The drawing under review shows one solid part. Ordinate dimensions are in mm from its lowest x, y, z. Round coordinates to 2 decimals unless told otherwise and drop trailing zeros. Order: outer loops, then holes, each group sorted by start corner. A loop starts at its lowest first (then second) coordinate and runs counter-clockwise, first axis right, second up.
1) Consider section B-B (z = 19.11). Give the boundary of the cut face in (x, y).
2) Consider section A-A (x = 1.4). Give the boundary of the cut face in (y, z).
3) To check wall thickness, follow L1, parallel to X at y = 1.1, z = 19.11; L2, parallel to Z at x = 43.91, y = 1.2; L3, parallel to Z at x = 2, y = 0.7. State the ranges of each line that lie inside material, in increasing order.
4) Clearance check with a flat-ended pin moving along its axis: P1, Ø1.4, axis at x = 1.4, z = 19.11, coming from the -Y side. State where the tip first meets the part, or that it passes through.
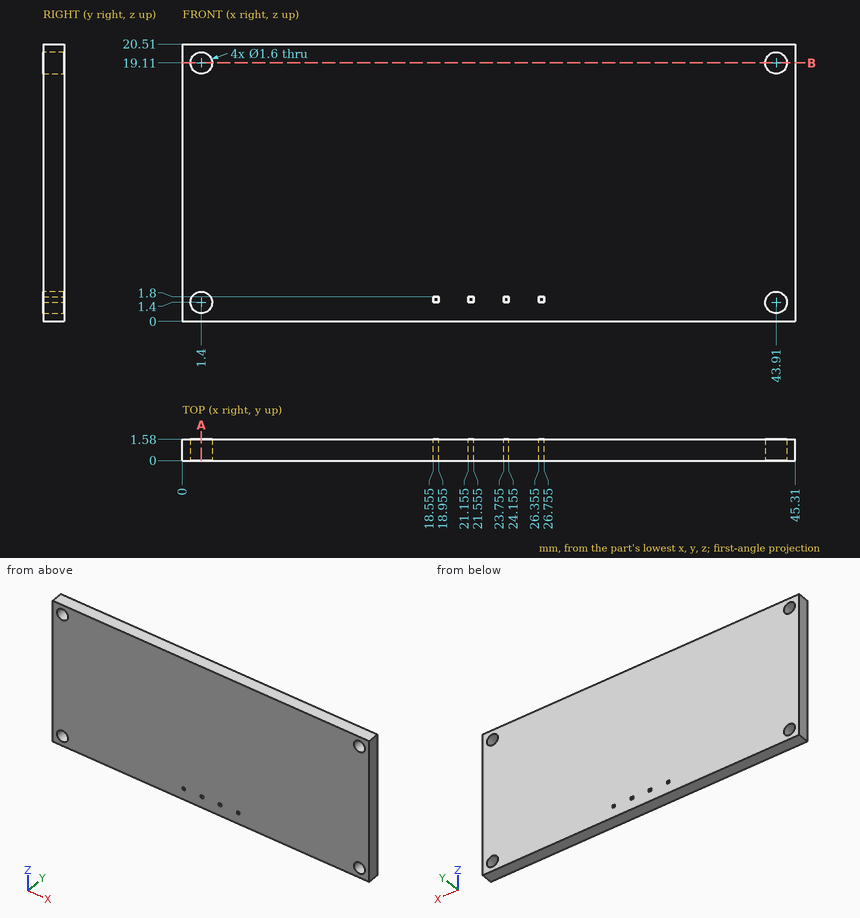
Answer below:
1. outline: (0, 0) - (0.6, 0) - (0.6, 1.58) - (0, 1.58) - close; (2.2, 0) - (43.11, 0) - (43.11, 1.58) - (2.2, 1.58) - close; (44.71, 0) - (45.31, 0) - (45.31, 1.58) - (44.71, 1.58) - close
2. outline: (0, 0) - (1.58, 0) - (1.58, 0.6) - (0, 0.6) - close; (0, 2.2) - (1.58, 2.2) - (1.58, 18.31) - (0, 18.31) - close; (0, 19.91) - (1.58, 19.91) - (1.58, 20.51) - (0, 20.51) - close
3. L1: x = 0 to 0.6, 2.2 to 43.11, 44.71 to 45.31
3. L2: z = 0 to 0.6, 2.2 to 18.31, 19.91 to 20.51
3. L3: z = 0 to 0.87, 1.93 to 18.58, 19.64 to 20.51
4. P1: passes through
